Answer from the drawing. Dimensions are ordinates in mm from the lowest x, y and z of the part. A direction names the side the tool comes from. Coordinates: 2 decimals unless noted, no trailing zeros. Order: outer loops, then holes, each group sorted by start corner. A loop starts at its lowest first (then second) coordinate and runs counter-clockwise, first axis right, second up.
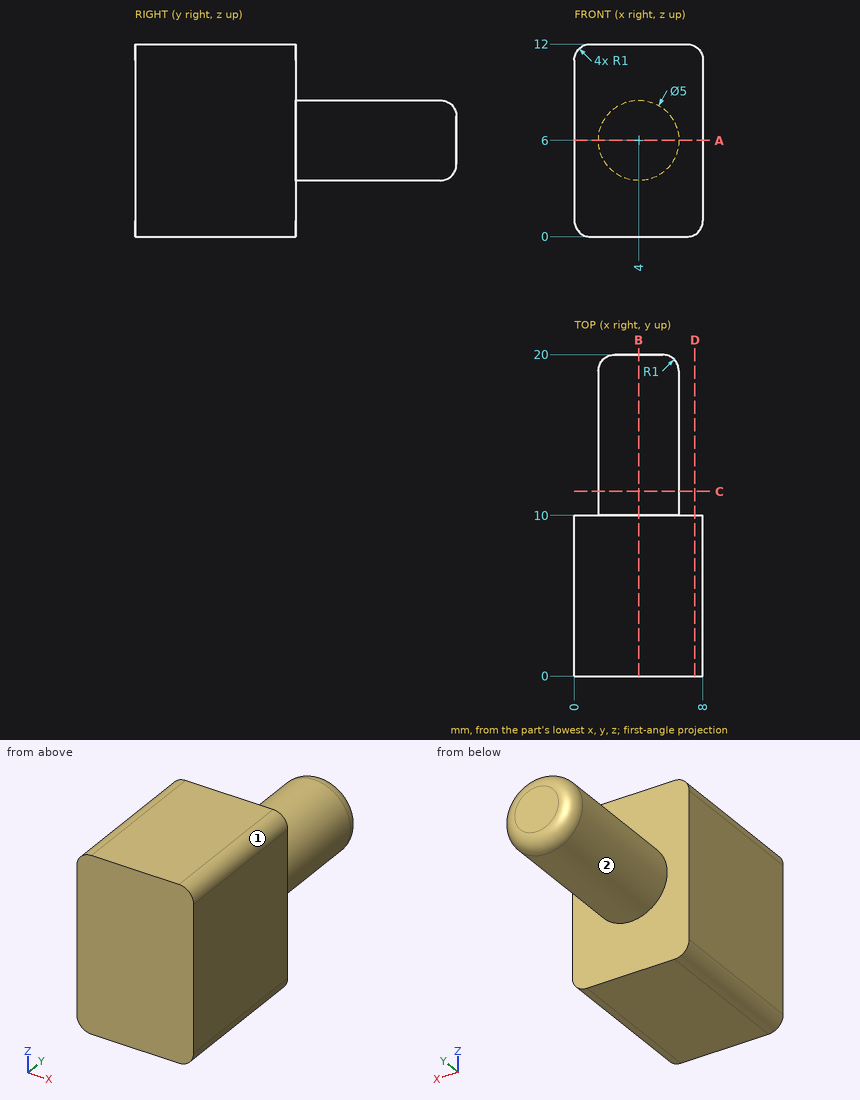
1) Section D-D (x = 7.5) is taken. Give the vertices of the cut face in (y, z).
2) Section C-C (y = 11.5) is taken. Give the vertices of the cut face in (x, z), then the cut area to 3 significant figures.
3) Section A-A (z = 6) is taken. Give the vertices of the cut face in (x, y).
4) Consider L1, parallel to Y at x = 3, z = 1; L2, parallel to X at y = 15.5, z = 4; L3, parallel to Z at x = 6, y = 11.75. Determine where each line is inside the solid, lowest interval first.
5) Each of these flat-tipped pins is pushed along its axis until it touches: P1, Ø2.5, axis at x = 3, z = 9, coming from the +Y side; P2, Ø3, axis at x = 2.5, z = 2, coming from the -Y side; P3, Ø4, axis at x = 2, y = 13, coming from the +Z side. Where does it stop, or does it pass through?
6) A tool of negligible diameter and unlimited length cuts with its end or side. For the marked faces 1 and 2, from which of +Z, -Z, +X, -X, +Y, -Y can it reach the whole face along a straight path? Write none if from no direction.
7) Section B-B (x = 4) is taken. Give the vertices of the cut face in (y, z).
Filled sheet:
1. outline: (0, 0.13) - (10, 0.13) - (10, 11.87) - (0, 11.87) - close
2. outline: circle Ø5 at (4, 6)
2. area: 19.6 mm2
3. outline: (0, 0) - (8, 0) - (8, 10) - (6.5, 10) - (6.5, 19) arc R1 ccw to (5.5, 20) - (2.5, 20) arc R1 ccw to (1.5, 19) - (1.5, 10) - (0, 10) - close
4. L1: y = 0 to 10
4. L2: x = 2.5 to 5.5
4. L3: z = 4.5 to 7.5
5. P1: stops at y = 19.91
5. P2: stops at y = 0
5. P3: stops at z = 8.5
6. face 1: +Z, +X, +Y, -Y
6. face 2: +Y
7. outline: (0, 0) - (10, 0) - (10, 3.5) - (19, 3.5) arc R1 ccw to (20, 4.5) - (20, 7.5) arc R1 ccw to (19, 8.5) - (10, 8.5) - (10, 12) - (0, 12) - close
